Autodesk Fusion 360 part; units mm, degrees
sketch "Sketch1" plane through (0, 0, 0) normal (0, 0, 1) x (1, 0, 0)
  line L0 (0, 0) -> (-118.5, 0) construction
  line L1 (-118.5, 0) -> (-118.5, 118.5) construction
  line L2 (-118.5, 118.5) -> (0, 118.5) construction
  line L3 (0, 118.5) -> (0, 0) construction
  line L4 (0, 0) -> (-26, 0)
  line L5 (-26, 0) -> (-26, 26)
  line L6 (-26, 26) -> (0, 26)
  line L7 (0, 26) -> (0, 0)
  dimension "d11" = 118.5
  dimension "d12" = 118.5
  dimension "d13" = 26
  dimension "d14" = 26
extrude "Extrude1" add sketch "Sketch1" along normal blind 16
sketch "Sketch2" plane through (0, 0, 16) normal (0, 0, 1) x (-1, 0, 0)
  line L0 (0, -26) -> (26, -26)
  line L1 (26, -26) -> (26, 0)
  line L2 (26, 0) -> (0, 0)
  line L3 (0, 0) -> (0, -26)
  circle A0 centre (6.3, -6.3) radius 2
  dimension "d17" = 4
  dimension "d18" = 6.3
  dimension "d19" = 6.3
extrude "Extrude2" cut sketch "Sketch2" against normal up to surface (16 mm away) contours A0
sketch "Sketch3" plane through (0, 0, 0) normal (0, 0, 1) x (1, 0, 0)
  line L0 (0, 0) -> (-118.5, 0) construction
  line L1 (-118.5, 0) -> (-118.5, 118.5) construction
  line L2 (-118.5, 118.5) -> (0, 118.5) construction
  line L3 (0, 118.5) -> (0, 0) construction
  line L4 (-118.5, 59.25) -> (0, 59.25) construction
  line L5 (-59.25, 118.5) -> (-59.25, 0) construction
  circle A0 centre (-59.25, 59.25) radius 66.5
  dimension "d22" = 118.5
  dimension "d23" = 118.5
  dimension "d24" = 133
extrude "Extrude3" cut sketch "Sketch3" along normal up to surface (16 mm away)
sketch "Sketch4" plane through (0, 0, 0) normal (0, 0, 1) x (1, 0, 0)
  line L0 (-8.0678, 11.4265) -> (-18.8511, 22.2099)
  arc A0 (-18.8511, 22.2099) -> (-22.2099, 18.8511) centre (-20.5305, 20.5305) ccw
  line L1 (-22.2099, 18.8511) -> (-11.4265, 8.0678)
  arc A1 (-11.4265, 8.0678) -> (-8.0678, 11.4265) centre (-9.7471, 9.7471) ccw
  line L2 (-8.0678, 8.0678) -> (-22.2099, 22.2099) construction
  circle A2 centre (-6.3, 6.3) radius 2
  dimension "d27" = 4.75
  dimension "d28" = 2.5
extrude "Extrude4" cut sketch "Sketch4" along normal up to surface (16 mm away) contours L0 A0 L1 A1
sketch "Sketch5" plane through (0, 0, 0) normal (0, 0, 1) x (1, 0, 0)
sketch "Sketch6" plane through (0, 0, 16) normal (0, 0, 1) x (-1, 0, 0)
  circle A0 centre (6.3, -6.3) radius 2
  line L0 (10.578, -13.9368) -> (8.0678, -11.4265)
  arc A1 (11.4265, -8.0678) -> (8.0678, -11.4265) centre (9.7471, -9.7471) ccw
  line L1 (11.4265, -8.0678) -> (13.9368, -10.578)
  arc A2 (26, -1.6593) -> (13.9368, -10.578) centre (59.25, -59.25) ccw
  line L2 (26, -1.6593) -> (26, 0)
  line L3 (26, 0) -> (0, 0)
  line L4 (0, 0) -> (0, -26)
  line L5 (0, -26) -> (1.6593, -26)
  arc A3 (10.578, -13.9368) -> (1.6593, -26) centre (59.25, -59.25) ccw
  line L6 (11.4265, -8.0678) -> (26, -0.8297)
  line L7 (26, -1.6593) -> (13.9368, -10.578)
  line L8 (13.9368, -10.578) -> (11.4265, -8.0678)
  line L9 (26, -1.6593) -> (26, -0.8297)
extrude "Extrude5" cut sketch "Sketch6" against normal up to surface (16 mm away) contours L1 A2 L2 L6 L8 L9
sketch "Sketch7" plane through (0, 0, 16) normal (0, 0, 1) x (-1, 0, 0)
  line L0 (11.4265, -8.0678) -> (26, -0.8297)
  line L1 (26, -0.8297) -> (26, 0)
  line L2 (26, 0) -> (0, 0)
  line L3 (0, 0) -> (0, -26)
  line L4 (0, -26) -> (1.6593, -26)
  arc A0 (10.578, -13.9368) -> (1.6593, -26) centre (59.25, -59.25) ccw
  line L5 (10.578, -13.9368) -> (8.0678, -11.4265)
  arc A1 (11.4265, -8.0678) -> (8.0678, -11.4265) centre (9.7471, -9.7471) ccw
  circle A2 centre (6.3, -6.3) radius 2
  line L6 (8.0678, -11.4265) -> (0.8297, -26)
  line L7 (0.8297, -26) -> (1.6593, -26)
  line L8 (1.6593, -26) -> (10.578, -13.9368)
  line L9 (10.578, -13.9368) -> (8.0678, -11.4265)
extrude "Extrude6" cut sketch "Sketch7" against normal up to surface (16 mm away) contours L4 A0 L5 L6 L7 L9
sketch "Sketch8" plane through (0, 0, 0) normal (1, 0, 0) x (0, 1, 0)
  line L0 (0, 0) -> (26, 0)
  line L1 (26, 0) -> (26, 16)
  line L2 (26, 16) -> (0, 16)
  line L3 (0, 16) -> (0, 0)
  circle A0 centre (18, 8) radius 1.625
  dimension "d39" = 3.25
  dimension "d40" = 18
extrude "Extrude7" cut sketch "Sketch8" along normal up to surface contours A0 end surface through (-8.0678, 11.4265, 16) normal (-0.895619, 0.444821, 0) offset 0
sketch "Sketch9" plane through (0, 0, 0) normal (1, 0, 0) x (0, 1, 0)
  circle A0 centre (18, 8) radius 1.625
  line L0 (0, 0) -> (26, 0)
  line L1 (26, 0) -> (26, 16)
  line L2 (26, 16) -> (0, 16)
  line L3 (0, 16) -> (0, 0)
  line L4 (21.25, 5.2) -> (14.75, 5.2)
  line L5 (14.75, 5.2) -> (14.75, 10.8)
  line L6 (14.75, 10.8) -> (21.25, 10.8)
  line L7 (21.25, 10.8) -> (21.25, 5.2)
  line L8 (21.25, 5.2) -> (14.75, 10.8) construction
  line L9 (14.75, 5.2) -> (21.25, 10.8) construction
  point P0 (18, 8)
  dimension "d46" = 6.5
  dimension "d47" = 5.6
extrude "Extrude8" cut sketch "Sketch9" along normal up to surface from surface at -2 contours L4 L5 L6 L7 end surface through (-8.0678, 11.4265, 16) normal (-0.895619, 0.444821, 0) offset 0
equation "fan_mount_hole_diameter = 4 mm"
equation "fan_mount_length = 26 mm"
equation "fan_mount_width = 16 mm"
equation "fan_mount_height = 26 mm"
equation "fan_inner_diameter = 115.2 mm"
equation "fan_mount_hole_edge_offset = 4.3 mm + ( fan_mount_hole_diameter / 2 )"
equation "fan_outer_mount_strut_width = 4.75 mm"
equation "fan_cove_radius = 66.5 mm"
equation "fan_mount_hole_cove_offset = 6 mm"
equation "fan_overall_width = 118.5 mm"
equation "d11 = fan_overall_width"
equation "d12 = fan_overall_width"
equation "d13 = fan_mount_length"
equation "d14 = fan_mount_height"
equation "d15 = fan_mount_width"
equation "d17 = fan_mount_hole_diameter"
equation "d18 = fan_mount_hole_edge_offset"
equation "d19 = fan_mount_hole_edge_offset"
equation "d22 = fan_overall_width"
equation "d23 = fan_overall_width"
equation "d24 = 2 * fan_cove_radius"
equation "d27 = fan_outer_mount_strut_width"
equation "d28 = ( fan_mount_hole_diameter / 2 ) + fan_strut_hole_offset"
equation "fan_strut_hole_offset = 0.5 mm"
equation "sharp_corner_fillet = 2 mm"
equation "bottom_hole_diameter = 3.25 mm"
equation "bottom_hole_edge_offset = 18 mm"
equation "d39 = bottom_hole_diameter"
equation "d40 = bottom_hole_edge_offset"
equation "bottom_screw_mount_nut_holder_width = 5.6 mm"
equation "bottom_screw_mount_nut_holder_length = 6.5 mm"
equation "bottom_screw_mount_nut_holder_bottom_offset = 2 mm"
equation "d46 = bottom_screw_mount_nut_holder_length"
equation "d47 = bottom_screw_mount_nut_holder_width"
For this review, take the finished solid that the model builds, in its own axes (mm). A direction names the side the tool comes from. Coordinates: 2 decimals unless noted, no trailing zeros. Write each loop counter-clockwise with the first axis right and the second up, starting at its lowest first coordinate (ties: lowest second). Pieces come first, ordered by that corner, then holes.
(1) For pin 1 Ø2 at (x, z) = (-7.5, 11.5) entering from +Y; pin 2 Ø8 at (x, z) = (-17, 13.5) entering from +Y; pin 3 Ø5 at (x, y) = (-8, 18.5) entering from -Z; pin 4 Ø4 at (y, z) = (6, 4.5) entering from -X, all flat-tipped, find the tip position at first contact; note any pin that passes through.
(2) Wall thickness on probe 1 along Y at (x, z) = (-6.3, 6.75); probe 2 along Z at (x, y) = (-0.95, 18) (3 decimals); probe 3 along X at (y, z) = (19, 2): over which ranges is each line inside the solid? List them lowest first.
(3) Add section B-B on y = 18. Give the boundary of the cut face in (x, z) (3 decimals).
(4) Add section C-C on z = 4.25. Give the boundary of the cut face in (x, y), then the cut area to 3 significant figures.
(5) The part is to be moulded in two halves that separate along Y. For faces 1 (the face through (-2, 18, 10)), 2 (the face through (0, 13, 8)), 3 (the face through (-0.4, 26, 7.9)), say which applies: +Y half, -Y half, draft (parallel to the pull), parting line (faces both ways), or undercut.
(6) Add section D-D on y = 6.3. Give the boundary of the cut face in (x, z).
(7) Add section A-A on z = 8. Count the separate pieces of the cut face and the enclosed holes in it, then the cut area to 3 significant figures.
(8) Tool access review of faces 4 (the face through (-5.866, 8.252, 8.112)), 5 (the face through (-4, 17, 10.8)): name each direction out of +Z, -Z, +X, -X, +Y, -Y from which nothing blocks a thin tool from reaching the whole face with its end or side.
Answer sheet:
1. pin 1: stops at y = 14.58
1. pin 2: stops at y = 7.29
1. pin 3: passes through
1. pin 4: stops at x = -19.62
2. probe 1: y = 0 to 4.3, 8.3 to 14.75
2. probe 2: z = 0 to 6.375, 9.625 to 16
2. probe 3: x = -4.31 to 0
3. outline: (-4.803, 0) - (0, 0) - (0, 6.375) - (-2, 6.375) - (-2, 5.2) - (-4.803, 5.2) - close; (-4.803, 10.8) - (-2, 10.8) - (-2, 9.625) - (0, 9.625) - (0, 16) - (-4.803, 16) - close
4. outline: (-26, 0) - (0, 0) - (0, 26) - (-0.83, 26) - (-8.07, 11.43) arc R2.37 cw to (-11.43, 8.07) - (-26, 0.83) - close; hole circle Ø4 at (-6.3, 6.3)
4. area: 233 mm2
5. face 1: undercut
5. face 2: draft
5. face 3: +Y half
6. outline: (-14.99, 0) - (-8.3, 0) - (-8.3, 16) - (-14.99, 16) - close; (-4.3, 0) - (0, 0) - (0, 16) - (-4.3, 16) - close
7. separate pieces: 2
7. enclosed holes: 1
7. area: 208 mm2
8. face 4: +Z, -Z
8. face 5: -X
